from build123d import *

# Parameters (mm, degrees)
SKETCH_1_R          = 6.791944052
SKETCH_1_R_2        = 3.995261207
EXTRUDE_1_DEPTH     = 40
CUT_EXTRUDE_1_DEPTH = 30
FILLET_1_R          = 50
SKETCH_3_W          = 68
SKETCH_3_H          = 60
CUT_EXTRUDE_2_DEPTH = 20
FILLET_2_R          = 30
FILLET_3_R          = 5
FILLET_4_R          = 5
CUT_EXTRUDE_3_DEPTH = 20


with BuildPart() as part:
    # ｽｹｯﾁ1 → ﾎﾞｽ - 押し出し1 (new body)
    with BuildSketch(Plane.XY):
        with BuildLine():
            Line((0, 0), (337.95498147, 0))
            ThreePointArc((337.95498147, 0), (357.931338385, -19.027804338), (339.897074223, -39.90548356))
            Line((339.897074223, -39.90548356), (79.782466467, -71.657339391))
            Line((79.782466467, -71.657339391), (65, -120))
            Line((65, -120), (0, -120))
            Line((0, -120), (0, 0))
        make_face()
        with Locations((337.95498147, -20)):
            Circle(SKETCH_1_R, mode=Mode.SUBTRACT)
        with Locations((37.95498147, -20)):
            Circle(SKETCH_1_R_2, mode=Mode.SUBTRACT)
    extrude(amount=EXTRUDE_1_DEPTH)

    # ｽｹｯﾁ2 → ｶｯﾄ - 押し出し1 (cut)
    with BuildSketch(Plane.XY.offset(40)):
        with BuildLine():
            Line((100, -6), (297.95498147, -6))
            ThreePointArc((297.95498147, -6), (313.853171972, -20.960808871), (299.884912284, -37.737756884))
            Line((299.884912284, -37.737756884), (101.211692948, -61.989541405))
            ThreePointArc((101.211692948, -61.989541405), (93.37115883, -59.550442937), (90, -52.063222842))
            Line((90, -52.063222842), (90, -16))
            ThreePointArc((90, -16), (92.928932188, -8.928932188), (100, -6))
        make_face()
    extrude(amount=-CUT_EXTRUDE_1_DEPTH, mode=Mode.SUBTRACT)

    # ﾌｨﾚｯﾄ1
    fillet_1_edges = [part.edges().sort_by_distance(p)[0] for p in [
        (79.782466467, -71.657339391, 20),
    ]]
    fillet(fillet_1_edges, radius=FILLET_1_R)

    # ｽｹｯﾁ3 → ｶｯﾄ - 押し出し2 (cut)
    with BuildSketch(Plane.XY.offset(40)):
        with Locations((34, -90)):
            Rectangle(SKETCH_3_W, SKETCH_3_H)
    extrude(amount=-CUT_EXTRUDE_2_DEPTH, mode=Mode.SUBTRACT)

    # ﾌｨﾚｯﾄ2
    fillet_2_edges = [part.edges().sort_by_distance(p)[0] for p in [
        (0, 0, 20),
    ]]
    fillet(fillet_2_edges, radius=FILLET_2_R)

    # ﾌｨﾚｯﾄ3
    fillet_3_edges = [part.edges().sort_by_distance(p)[0] for p in [
        (68, -60, 30),
    ]]
    fillet(fillet_3_edges, radius=FILLET_3_R)

    # ﾌｨﾚｯﾄ4
    fillet_4_edges = [part.edges().sort_by_distance(p)[0] for p in [
        (0, -120, 10),
    ]]
    fillet(fillet_4_edges, radius=FILLET_4_R)

    # ｽｹｯﾁ4 → ｶｯﾄ - 押し出し3 (cut)
    with BuildSketch(Plane.XY.offset(40)):
        with BuildLine():
            Line((78.036982516, 0), (58.355302576, -38.576774086))
            ThreePointArc((58.355302576, -38.576774086), (50.146919618, -48.212517196), (38.476348343, -53.113829488))
            Line((38.476348343, -53.113829488), (0, -53.113829488))
            Line((0, -53.113829488), (0, 0))
            Line((0, 0), (78.036982516, 0))
        make_face()
    extrude(amount=-CUT_EXTRUDE_3_DEPTH, mode=Mode.SUBTRACT)


solid = part.part
Read the model definition and answer for the solid it produces. Units are mm, in the model's axes. A direction names the side the tool comes from. Coordinates: 2 decimals unless noted, no trailing zeros. Loops run counter-clockwise (first coordinate to the right, second up) from the corner with the lowest first, then second, coordinate; pieces in that order, holes last. Notation, with made-up numbers: (53.5, 60.5) -> (76.5, 60.5) arc R20 cw to (76.5, 98.5) -> close; hole circle Ø8 at (61.5, 20.5). An arc over 180 degrees is marked (long way). Write item = value, one per line. Start each with the question number.
1) The part is cut by section B-B, the plane y = -20. Determine the outline of the cut face in (x, z), plus the area to 3 significant figures.
2) For faces 4 (the face through (68, -88, 30)), 5 (the face through (20, -53.114, 30)), 6 (the face through (86.28, -78.78, 20.28)), 7 (the face through (198, -6, 25)), determine the directions among +Z, -Z, +X, -X, +Y, -Y from which every point of the face is accessible in a straight line to the end or side of a thin tool.
3) The mould has two halves that part along X. Classify faces 1 (the face through (357.906, -18.602, 19.72)), 2 (the face through (344.433, -17.96, 19.72)), 3 (the face through (180, -55, 40)): pulls with the +X half, pulls with the -X half, needs draft (parallel to the pull), parting line crosses it, or undercut.
4) Given P1, Ø13, axis at x = 37.95, y = -20, coming from the +Z side; P2, Ø10, axis at x = 27, z = 28.5, coming from the -Y side; P3, Ø22, axis at y = -93, z = 26, coming from the -X side; P4, Ø5, axis at x = 227, y = -44, coming from the +Z side, each flat-ended and moving along its own axis, determine where each tip first touches the part or whether it passes through.
5) The part is cut by section C-C, the plane x = 254.5. Determine the outline of the cut face in (y, z).
6) Find the intervals of material crossed by L1, parallel to Z at x = 24.5, y = -79.5; L2, parallel to Y at x = 96.5, z = 19; L3, parallel to Y at x = 128, z = 12, in increasing order. Write a range as from..to.
7) The part is cut by section D-D, the plane y = -93.5. Determine the outline of the cut face in (x, z).
8) The part is cut by section A-A, the plane z = 27. Determine the outline of the cut face in (x, y), plus the area to 3 significant figures.
Result:
q1.outline = (1.72, 0) -> (33.96, 0) -> (33.96, 20) -> (1.72, 20) -> close; (41.95, 0) -> (331.16, 0) -> (331.16, 40) -> (313.77, 40) -> (313.77, 10) -> (90, 10) -> (90, 40) -> (67.83, 40) -> (67.83, 20) -> (41.95, 20) -> close; (344.75, 0) -> (357.95, 0) -> (357.95, 40) -> (344.75, 40) -> close
q1.area = 5,510 mm²
q2.face_4 = +Z, -X, -Y
q2.face_5 = +Z, -X, +Y
q2.face_6 = +Z, -Z, +X, -Y
q2.face_7 = +Z
q3.face_1 = pulls with the +X half
q3.face_2 = undercut
q3.face_3 = needs draft
q4.P1 = 20
q4.P2 = -60
q4.P3 = 0
q4.P4 = 10
q5.outline = (-50.33, 0) -> (0, 0) -> (0, 40) -> (-6, 40) -> (-6, 10) -> (-43.28, 10) -> (-43.28, 40) -> (-50.33, 40) -> close
q6.L1 = 0..20
q6.L2 = -72.26..-61.43, -6.63..0
q6.L3 = -65.77..-58.72, -6..0
q7.outline = (0, 0) -> (74.15, 0) -> (74.15, 40) -> (68, 40) -> (68, 20) -> (0, 20) -> close
q8.outline = (0, -60) -> (63, -60) arc R5 cw to (68, -65) -> (68, -110.19) -> (70.28, -102.73) arc R50 cw to (112.04, -67.72) -> (339.9, -39.91) arc R20 ccw to (337.95, 0) -> (78.04, 0) -> (58.36, -38.58) arc R27.32 cw to (38.48, -53.11) -> (0, -53.11) -> close; hole (90, -52.06) arc R10 ccw to (101.21, -61.99) -> (299.88, -37.74) arc R15.93 ccw to (297.95, -6) -> (100, -6) arc R10 ccw to (90, -16) -> close; hole circle Ø13.58 at (337.95, -20)
q8.area = 7,240 mm²
